Part print with two shaded views. Sizes in mm from the minimum x, y, z corner. Give positions to 0.01 mm unless a question says otherwise; leave off trailing zeros. Order: outer loops, then holes, each group sorted by start corner. A loop starts at its lowest first (then second) coordinate and runs counter-clockwise, first axis right, second up. Notation, with made-up numbers: M 86,6 L 121,6 A17 cw 121,22 Z; hole C 24,24 d6. An arc over 180 degrees is marked long. Return JSON: item names as keys, results as strings.
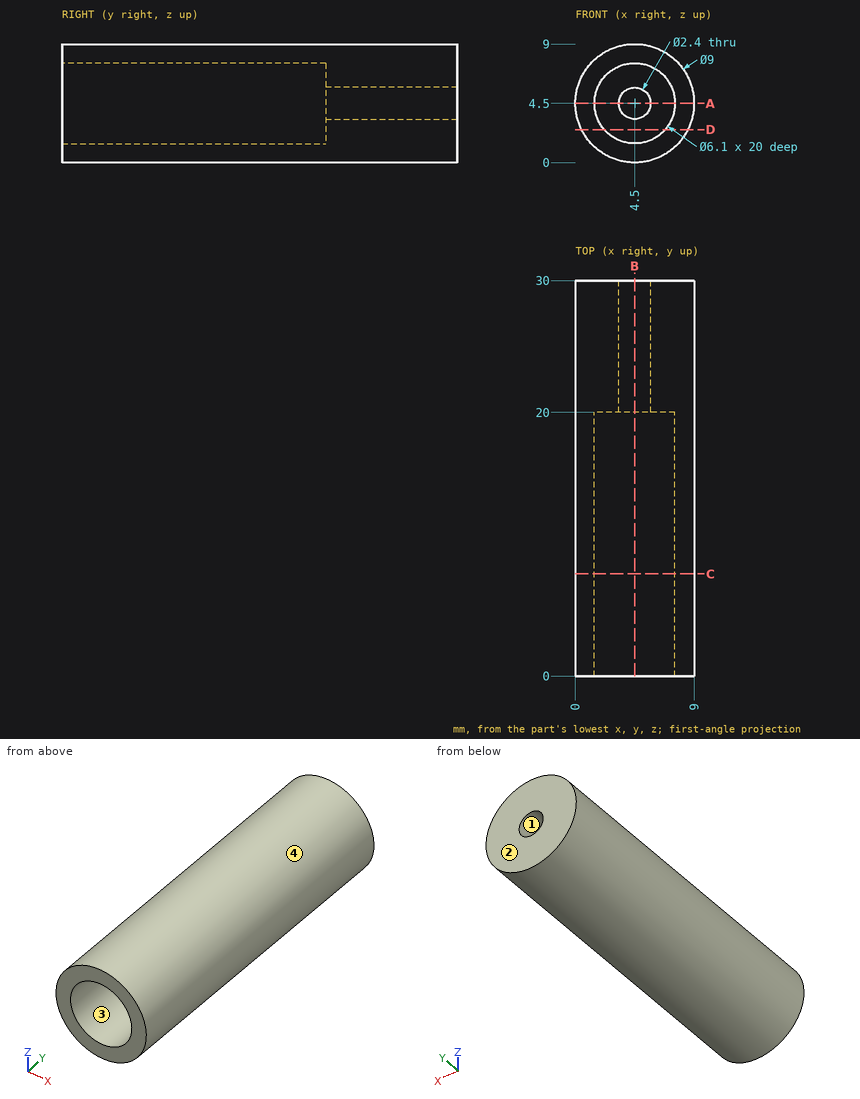
Q1. Band-saw the part on D-D (z = 2.5). Give the cut face in (x, y), then the cut area to 3 significant figures.
Established:
{"outline": "M 0.47,0 L 2.2,0 L 2.2,20 L 6.8,20 L 6.8,0 L 8.53,0 L 8.53,30 L 0.47,30 Z", "area": "150 mm²"}
Q2. Band-saw the part on C-C (y = 7.75). Give the cut face in (x, z).
Established:
{"outline": "C 4.5,4.5 d9; hole C 4.5,4.5 d6.1"}
Q3. Two-plate mould, pull along Z, no slides. Class the marked faces 1, 2, 3 and 4: +Z half, -Z half, draft (parallel to the pull), parting line (faces both ways), or undercut.
Established:
{"face 1": "undercut", "face 2": "draft", "face 3": "undercut", "face 4": "parting line"}
Q4. Band-saw the part on B-B (x = 4.5). Give the cut face in (y, z).
Established:
{"outline": "M 0,0 L 30,0 L 30,3.3 L 20,3.3 L 20,1.45 L 0,1.45 Z; M 0,7.55 L 20,7.55 L 20,5.7 L 30,5.7 L 30,9 L 0,9 Z"}
Q5. Pin check, flat tips, straight feed: pin 1 (1.4 mm diameter, centred on x = 4.5, z = 4.5, fed in from +Y); pin 2 (1.5 mm diameter, centred on x = 7.5, y = 4.5, fed in from -Z); pin 3 (2 mm diameter, centred on y = 16, z = 7.5, fed in from +X). Stop position of each tip, or through.
Established:
{"pin 1": "passes through", "pin 2": "stops at z = 0.6", "pin 3": "stops at x = 8.53"}
Q6. Probe line 1 along X through (y, z) = (24.5, 4.5); line 2 along X through (y, z) = (9.5, 4.5); line 3 along Z through (x, y) = (2.75, 15.75). List the from-to ranges inside material, lowest first.
Established:
{"line 1": "x = 0 to 3.3, 5.7 to 9", "line 2": "x = 0 to 1.45, 7.55 to 9", "line 3": "z = 0.35 to 2, 7 to 8.65"}
Q7. Band-saw the part on A-A (z = 4.5). Give the cut face in (x, y), then the cut area to 3 significant figures.
Established:
{"outline": "M 0,0 L 1.45,0 L 1.45,20 L 3.3,20 L 3.3,30 L 0,30 Z; M 5.7,20 L 7.55,20 L 7.55,0 L 9,0 L 9,30 L 5.7,30 Z", "area": "124 mm²"}
